The listing builds one solid part. Answer for the finished solid, in the listing's coordinates (mm). A direction names the side the tool comes from. Give positions to 0.01 mm unless a question says otherwise; leave off trailing zeros. Write each loop counter-clockwise with the first axis right and the second up, starting at its lowest first coordinate (ties: lowest second). Pieces come first, ordered by that corner, then holes. Notation, with made-up numbers: (25.25, -10) - (79.25, -10) arc R16 cw to (79.25, 14) - close; hole circle Ø6 at (84.25, 57). An arc over 180 degrees is marked (long way). One line per question, with ' | ' between items. Start each with the question number.
1. A cutting plane is placed at A-A (x = 0). Determine the outline of the cut face in (y, z).
2. Given P1, Ø8, axis at y = -6.5, z = 22, coming from the -X side; P2, Ø5, axis at x = 35.5, y = -25, coming from the +Z side; P3, Ø3, axis at x = -33, y = -16.5, coming from the -Z side, each flat-ended and moving along its own axis, determine where each tip first touches the part or whether it passes through.
3. A cutting plane is placed at B-B (y = 0). Determine the outline of the cut face in (x, z).
4. The mould has two halves that part along X. Classify faces 1 (the face through (-0.439, 33.863, 0.626)), 2 (the face through (-1.97, -54.06, 0.63)), 3 (the face through (0, 0, 38.1)): +X half, -X half, draft (parallel to the pull), parting line (faces both ways), or undercut.
5. A cutting plane is placed at C-C (z = 3.5). Determine the outline of the cut face in (x, y).
6. For faces 4 (the face through (-2.08, -9.367, 19.427)), 5 (the face through (-1, -3, 0)), determine the directions among +Z, -Z, +X, -X, +Y, -Y from which every point of the face is accessible in a straight line to the end or side of a thin tool.
7. Find the intervals of material crossed by L1, parallel to Z at x = 10, y = -34.5; L2, parallel to Y at x = 0, z = 31; L3, parallel to X at y = -5.5, z = 33.5, in increasing order. Write a range as from..to.
8. A cutting plane is placed at D-D (x = -40). Determine the outline of the cut face in (y, z).
```python
from build123d import *

# Parameters (mm, degrees)
F0_R     = 54.0947036541
F1_DEPTH = 1.27
F2_R     = 36.4799484266
F3_DEPTH = 25.4
F4_R     = 9.5951765944
F5_DEPTH = 38.1


# Not quite as in the source:
# - the program builds the solid bodies; features that only make, move or delete a surface that nothing else refers to are left out


with BuildPart() as f1:
    # F0 (on Top) → F1 (new body)
    with BuildSketch(Plane.XY):
        Circle(F0_R)
    extrude(amount=F1_DEPTH)

    # F2 (on Top) → F3 (cut)
    with BuildSketch(Plane.XY):
        with Locations((0, 70.3405514359)):
            Circle(F2_R)
    extrude(amount=F3_DEPTH, mode=Mode.SUBTRACT)

    # F4 (on Top) → F5 (join)
    with BuildSketch(Plane.XY):
        Circle(F4_R)
    extrude(amount=F5_DEPTH)


solid = f1.part
```
Determined:
1) outline: (-54.09, 0) - (33.86, 0) - (33.86, 1.27) - (9.6, 1.27) - (9.6, 38.1) - (-9.6, 38.1) - (-9.6, 1.27) - (-54.09, 1.27) - close
2) P1: x = -9.26 | P2: z = 1.27 | P3: z = 0
3) outline: (-54.09, 0) - (54.09, 0) - (54.09, 1.27) - (9.6, 1.27) - (9.6, 38.1) - (-9.6, 38.1) - (-9.6, 1.27) - (-54.09, 1.27) - close
4) face 1: undercut | face 2: parting line | face 3: draft
5) outline: circle Ø19.19 at (0, 0)
6) face 4: +Z | face 5: -Z, +X, -X, +Y, -Y
7) L1: 0..1.27 | L2: -9.6..9.6 | L3: -7.86..7.86
8) outline: (-36.42, 0) - (36.42, 0) - (36.42, 1.27) - (-36.42, 1.27) - close
